```python
from build123d import *

# Parameters (mm, degrees)
SKETCH2_R            = 27.5
BOSS_EXTRUDE1_DEPTH  = 50
SKETCH3_R            = 26.75
CUT_EXTRUDE1_DEPTH   = 51
SKETCH7_R            = 18.25
BOSS_EXTRUDE3_DEPTH  = 50
SKETCH8_R            = 17.5
CUT_EXTRUDE3_DEPTH   = 51
SKETCH9_W            = 59.961193285
SKETCH9_H            = 28.516087398
CUT_EXTRUDE4_DEPTH   = 51
SKETCH10_W           = 0.75
SKETCH10_H           = 12.5
BOSS_EXTRUDE4_DEPTH  = 50
BOSS_EXTRUDE5_DEPTH  = 5
BOSS_EXTRUDE6_DEPTH  = 6.5
SKETCH12_W           = 14
SKETCH12_H           = 20
SKETCH12_W_2         = 20
SKETCH12_H_2         = 14
CUT_EXTRUDE6_DEPTH   = 15
SKETCH14_W           = 14
SKETCH14_H           = 20
CUT_EXTRUDE7_DEPTH   = 45
SKETCH15_W           = 16.605878589
SKETCH15_H           = 22.2356131
CUT_EXTRUDE8_DEPTH   = 15
BOSS_EXTRUDE8_DEPTH  = 4.5
BOSS_EXTRUDE9_DEPTH  = 2
BOSS_EXTRUDE10_DEPTH = 2
BOSS_EXTRUDE15_DEPTH = 24
BOSS_EXTRUDE17_DEPTH = 10
SKETCH26_W           = 5
SKETCH26_H           = 18
BOSS_EXTRUDE18_DEPTH = 10
SKETCH27_W           = 8.5
SKETCH27_H           = 14
BOSS_EXTRUDE19_DEPTH = 5


with BuildPart() as part:
    # Sketch2 → Boss-Extrude1 (new body)
    with BuildSketch(Plane(origin=(0, 0, 0), x_dir=(1, 0, 0), z_dir=(0, 1, 0))):
        Circle(SKETCH2_R)
    extrude(amount=BOSS_EXTRUDE1_DEPTH)

    # Sketch3 → Cut-Extrude1 (cut, through all)
    with BuildSketch(Plane(origin=(0, 50, 0), x_dir=(1, 0, 0), z_dir=(0, 1, 0))):
        Circle(SKETCH3_R)
    extrude(amount=-CUT_EXTRUDE1_DEPTH, mode=Mode.SUBTRACT)


with BuildPart() as body_2:
    # Sketch7 → Boss-Extrude3 (new body)
    with BuildSketch(Plane(origin=(0, 50, 0), x_dir=(1, 0, 0), z_dir=(0, 1, 0))):
        Circle(SKETCH7_R)
    extrude(amount=-BOSS_EXTRUDE3_DEPTH)

    # Sketch8 → Cut-Extrude3 (cut, through all)
    with BuildSketch(Plane(origin=(0, 50, 0), x_dir=(1, 0, 0), z_dir=(0, 1, 0))):
        Circle(SKETCH8_R)
    extrude(amount=-CUT_EXTRUDE3_DEPTH, mode=Mode.SUBTRACT)


with BuildPart() as cut_extrude4_tool:
    # Sketch9 → Cut-Extrude4 (new body, through all)
    with BuildSketch(Plane(origin=(0, 50, 0), x_dir=(1, 0, 0), z_dir=(0, 1, 0))):
        with Locations((-0.477134602, -14.258043699)):
            Rectangle(SKETCH9_W, SKETCH9_H)
    extrude(amount=-CUT_EXTRUDE4_DEPTH)


with BuildPart() as part_1:
    add(part.part)

    # Cut-Extrude4: cut by cut_extrude4_tool
    add(cut_extrude4_tool.part, mode=Mode.SUBTRACT)



with BuildPart() as body_2_1:
    add(body_2.part)

    # Cut-Extrude4: cut by cut_extrude4_tool
    add(cut_extrude4_tool.part, mode=Mode.SUBTRACT)


with BuildPart() as part_2:
    add(part_1.part)

    add(body_2_1.part)  # Boss-Extrude4 merges body 2
    # Sketch10 → Boss-Extrude4 (add)
    with BuildSketch(Plane(origin=(0, 50, 0), x_dir=(1, 0, 0), z_dir=(0, 1, 0))):
        with Locations((-27.125, -6.25)):
            Rectangle(SKETCH10_W, SKETCH10_H)
        with Locations((-17.875, -6.25)):
            Rectangle(SKETCH10_W, SKETCH10_H)
        with Locations((17.875, -6.25)):
            Rectangle(SKETCH10_W, SKETCH10_H)
        with Locations((27.125, -6.25)):
            Rectangle(SKETCH10_W, SKETCH10_H)
    extrude(amount=-BOSS_EXTRUDE4_DEPTH)

    # Sketch11 → Boss-Extrude5 (add)
    with BuildSketch(Plane(origin=(0, 50, 0), x_dir=(1, 0, 0), z_dir=(0, 1, 0))):
        with BuildLine():
            Line((16.760723177, 7.220848882), (24.236408431, 11.320733473))
            ThreePointArc((24.236408431, 11.320733473), (26.114042444, 5.798214142), (26.75, 0))
            Line((26.75, 0), (26.75, -12.5))
            Line((26.75, -12.5), (18.25, -12.5))
            Line((18.25, -12.5), (18.25, 0))
            ThreePointArc((18.25, 0), (17.873803428, 3.686414384), (16.760723177, 7.220848882))
        make_face()
    extrude(amount=-BOSS_EXTRUDE5_DEPTH)

    # Sketch13 → Boss-Extrude6 (add)
    with BuildSketch(Plane.XZ):
        with BuildLine():
            Line((18.25, 0), (18.25, 12.5))
            Line((18.25, 12.5), (26.75, 12.5))
            Line((26.75, 12.5), (26.75, 0))
            ThreePointArc((26.75, 0), (26.114042444, -5.798214142), (24.236408431, -11.320733473))
            Line((24.236408431, -11.320733473), (16.760723177, -7.220848882))
            ThreePointArc((16.760723177, -7.220848882), (17.873803428, -3.686414384), (18.25, 0))
        make_face()
    extrude(amount=-BOSS_EXTRUDE6_DEPTH)

    # Sketch12 → Cut-Extrude6 (cut)
    with BuildSketch(Plane(origin=(27.5, 0, 0), x_dir=(0, 0, -1), z_dir=(1, 0, 0))):
        with Locations((-0.5, 35)):
            Rectangle(SKETCH12_W, SKETCH12_H)
        with Locations((2.5, 13.5)):
            Rectangle(SKETCH12_W_2, SKETCH12_H_2)
    extrude(amount=-CUT_EXTRUDE6_DEPTH, mode=Mode.SUBTRACT)

    # Sketch14 → Cut-Extrude7 (cut)
    with BuildSketch(Plane.XY.offset(12.5)):
        with Locations((0, 25)):
            Rectangle(SKETCH14_W, SKETCH14_H)
    extrude(amount=-CUT_EXTRUDE7_DEPTH, mode=Mode.SUBTRACT)

    # Sketch15 → Cut-Extrude8 (cut)
    with BuildSketch(Plane.ZY.offset(27.5)):
        with Locations((15.802939295, 43.11780655)):
            Rectangle(SKETCH15_W, SKETCH15_H)
    extrude(amount=-CUT_EXTRUDE8_DEPTH, mode=Mode.SUBTRACT)

    # Sketch17 → Boss-Extrude8 (add)
    with BuildSketch(Plane(origin=(0, 25, 0), x_dir=(1, 0, 0), z_dir=(0, 1, 0))):
        with BuildLine():
            Line((26.720778432, 6.5), (17.053225501, 6.5))
            ThreePointArc((17.053225501, 6.5), (17.948312809, 3.304628164), (18.25, 0))
            Line((18.25, 0), (18.25, -7.5))
            Line((18.25, -7.5), (27.5, -7.5))
            Line((27.5, -7.5), (27.5, 0))
            ThreePointArc((27.5, 0), (27.304499692, 3.273270011), (26.720778432, 6.5))
        make_face()
    extrude(amount=-BOSS_EXTRUDE8_DEPTH)

    # Sketch18 → Boss-Extrude9 (add)
    with BuildSketch(Plane.XZ.offset(-35)):
        with BuildLine():
            Line((-7, -16.854153791), (-7, -25.817871717))
            ThreePointArc((-7, -25.817871717), (0, -26.75), (7, -25.817871717))
            Line((7, -25.817871717), (7, -16.854153791))
            ThreePointArc((7, -16.854153791), (0, -18.25), (-7, -16.854153791))
        make_face()
    extrude(amount=-BOSS_EXTRUDE9_DEPTH)

    # Sketch19 → Boss-Extrude10 (add)
    with BuildSketch(Plane(origin=(0, 15, 0), x_dir=(1, 0, 0), z_dir=(0, 1, 0))):
        with BuildLine():
            Line((7, 25.817871717), (7, 16.854153791))
            ThreePointArc((7, 16.854153791), (0, 18.25), (-7, 16.854153791))
            Line((-7, 16.854153791), (-7, 25.817871717))
            ThreePointArc((-7, 25.817871717), (0, 26.75), (7, 25.817871717))
        make_face()
    extrude(amount=-BOSS_EXTRUDE10_DEPTH)

    # Sketch24 → Boss-Extrude15 (add)
    with BuildSketch(Plane(origin=(0, 37, 0), x_dir=(1, 0, 0), z_dir=(0, 1, 0))):
        with BuildLine():
            Line((8.47493115, 25.37199326), (8.47493115, 16.162859957))
            ThreePointArc((8.47493115, 16.162859957), (7.745182071, 16.524970641), (7, 16.854153791))
            Line((7, 16.854153791), (7, 25.817871717))
            ThreePointArc((7, 25.817871717), (7.740676678, 25.605554565), (8.47493115, 25.37199326))
        make_face()
    extrude(amount=-BOSS_EXTRUDE15_DEPTH)

    # Sketch25 → Boss-Extrude17 (add)
    with BuildSketch(Plane(origin=(27.5, 0, 0), x_dir=(0, 0, -1), z_dir=(1, 0, 0))):
        Polygon((-7.5, 45), (-12.5, 45), (-12.5, 25), (-12.5, 20.5), (-7.5, 20.5), (-7.5, 25), align=None)
    extrude(amount=-BOSS_EXTRUDE17_DEPTH)

    # Sketch26 → Boss-Extrude18 (add)
    with BuildSketch(Plane.ZY.offset(27.5)):
        with Locations((10, 23)):
            Rectangle(SKETCH26_W, SKETCH26_H)
    extrude(amount=-BOSS_EXTRUDE18_DEPTH)

    # Sketch27 → Boss-Extrude19 (add)
    with BuildSketch(Plane.XY.offset(12.5)):
        with Locations((22.5, 13.5)):
            Rectangle(SKETCH27_W, SKETCH27_H)
    extrude(amount=-BOSS_EXTRUDE19_DEPTH)


solid = part_2.part
```
The model under review builds one solid part; all positions refer to its coordinate system, in mm. A direction names the side the tool comes from. Give positions to 0.01 mm unless a question says otherwise; leave off trailing zeros. Write each loop counter-clockwise with the first axis right and the second up, starting at its lowest first coordinate (ties: lowest second). Pieces come first, ordered by that corner, then holes. Notation, with made-up numbers: (48.5, -22) - (57.5, -22) arc R21 ccw to (57.5, 13) - close; hole circle Ø4 at (89, 27). An arc over 180 degrees is marked (long way). Answer in a Markdown table with one row per item. Add a question column.
1. We need section B-B on x = 0. Write out the cut boundary in (y, z), then the cut area to 3 significant figures.
2. We need section D-D on z = 10.5. Write out the cut boundary in (x, y).
3. Tool access review of faces 4 (the flat face through (1, 13, -22)), 5 (the flat face through (22, 20.5, 0)), 6 (the flat face through (8.475, 25, -21)): name each direction out of +Z, -Z, +X, -X, +Y, -Y from which nothing blocks a thin tool from reaching the whole face with its end or side.
4. Draft analysis for pull direction X (two halves, no side actions). For faces 1 (the flat face through (-23, 32, 10)), 2 (the cylindrical face through (-11.01, 25.35, -24.38)), 3 (the cylindrical face through (-8.84, 24.65, -26.04)), state which applies: +X half, -X half, draft (parallel to the pull), parting line (faces both ways), or undercut.
5. We need section C-C on y = 40. Write out the cut boundary in (x, z).
6. Wall thickness on line 1 along X through (y, z) = (7, -16); line 2 along X through (y, z) = (5.5, -6); line 3 along X through (y, z) = (9, -13.5): over which ranges is each line inside the solid? List them lowest first. Write a range as [from, to].
7. Insertion check: P1, Ø3, axis at y = 14, z = -15.5, coming from the -X side; P2, Ø1, axis at x = -1, y = 12.5, coming from the +Z side; P3, Ø3, axis at y = 22.5, z = -19.5, coming from the +X side; P4, Ø3, axis at x = 4, z = -13.5, coming from the -Y side. Each pin has a flat end and moves straight along its axis. Give the tip position at first contact, or say it passes through.
8. We need section A-A on z = 4.5. Write out the cut boundary in (x, y).
Ans:
| question | item | result |
|---|---|---|
| 1 | outline | (0, -27.5) - (15, -27.5) - (15, -17.5) - (0, -17.5) - (0, -18.25) - (13, -18.25) - (13, -26.75) - (0, -26.75) - close; (35, -27.5) - (50, -27.5) - (50, -26.75) - (37, -26.75) - (37, -18.25) - (50, -18.25) - (50, -17.5) - (35, -17.5) - close |
| 1 | area | 79.0 mm^2 |
| 2 | outline | (-27.5, 0) - (-26.75, 0) - (-26.75, 14) - (-18.25, 14) - (-18.25, 0) - (-17.5, 0) - (-17.5, 32) - (-27.5, 32) - close; (17.5, 0) - (27.5, 0) - (27.5, 50) - (17.5, 50) - close |
| 3 | face 4 | -Y |
| 3 | face 5 | +X |
| 3 | face 6 | +Y, -Y |
| 4 | face 1 | draft |
| 4 | face 2 | undercut |
| 4 | face 3 | parting line |
| 5 | outline | (-27.5, 0) arc R27.5 ccw to (26.72, -6.5) - (25.95, -6.5) arc R26.75 cw to (-26.75, 0) - (-26.75, 7.5) - (-27.5, 7.5) - close; (-18.25, 0) arc R18.25 ccw to (17.05, -6.5) - (16.25, -6.5) arc R17.5 cw to (-17.5, 0) - (-17.5, 7.5) - (-18.25, 7.5) - close; (17.5, 7.5) - (27.5, 7.5) - (27.5, 12.5) - (17.5, 12.5) - close |
| 6 | line 1 | x = [-22.37, -21.44], [-8.78, -7.09], [7.09, 8.78], [21.44, 22.37] |
| 6 | line 2 | x = [-26.84, -26.07], [-17.24, -16.44], [16.44, 26.84] |
| 6 | line 3 | x = [-23.96, -23.09], [-12.28, -11.14], [11.14, 12.28], [23.09, 23.96] |
| 7 | P1 | stops at x = -23.67 |
| 7 | P2 | stops at z = -17.44 |
| 7 | P3 | stops at x = 20.79 |
| 7 | P4 | passes through |
| 8 | outline | (-27.5, 0) - (-26.75, 0) - (-26.75, 50) - (-27.5, 50) - close; (-18.25, 0) - (-17.5, 0) - (-17.5, 50) - (-18.25, 50) - close; (17.5, 0) - (27.5, 0) - (27.5, 6.5) - (17.5, 6.5) - close; (17.5, 20.5) - (27.5, 20.5) - (27.5, 25) - (17.5, 25) - close; (17.5, 45) - (27.5, 45) - (27.5, 50) - (17.5, 50) - close |
